from build123d import *

# Parameters (mm, degrees)
F0_W     = 70
F0_H     = 70
F0_R     = 1.1
F0_R_2   = 5.75
F1_DEPTH = 1.5
F3_DEPTH = 1.5


with BuildPart() as f1:
    # F0 (on Top) → F1 (new body)
    with BuildSketch(Plane.XY):
        Rectangle(F0_W, F0_H)
        with Locations((-20.071068, -5.384776)):
            Circle(F0_R, mode=Mode.SUBTRACT)
        with Locations((-31.384776, 5.928932)):
            Circle(F0_R, mode=Mode.SUBTRACT)
        with Locations((-4.868272, 21.131728)):
            Circle(F0_R_2, mode=Mode.SUBTRACT)
        with Locations((-5.928932, 31.384776)):
            Circle(F0_R, mode=Mode.SUBTRACT)
        with Locations((5.384776, 20.071068)):
            Circle(F0_R, mode=Mode.SUBTRACT)
    extrude(amount=F1_DEPTH)

    # F2 (on face) → F3 (cut, through all)
    with BuildSketch(Plane.XY.offset(1.5)):
        Polygon((-35, 35), (-35, 6.556349), (-6.556349, 35), align=None)
        Polygon((-20.857864, -8.84062), (-35, 5.301515), (-35, -35), (-15, -35), (-15, -8.84062), align=None)
    extrude(amount=-F3_DEPTH, mode=Mode.SUBTRACT)


solid = f1.part
For this review, take the finished solid that the model builds, in its own axes (mm). A direction names the side the tool comes from. Give positions to 0.01 mm unless a question says otherwise; leave off trailing zeros. Order: outer loops, then holes, each group sorted by start corner. A loop starts at its lowest first (then second) coordinate and runs counter-clockwise, first axis right, second up. Notation, with made-up numbers: (8.25, 88) -> (37.25, 88) arc R25 cw to (37.25, 107) -> close; hole circle Ø5 at (0.25, 19). An arc over 180 degrees is marked (long way). Write item = value, one per line.
1) We need section A-A, the plane y = 24. Give the boundary of the cut face in (x, z).
Findings:
outline = (-17.56, 0) -> (-9.85, 0) -> (-9.85, 1.5) -> (-17.56, 1.5) -> close; (0.12, 0) -> (35, 0) -> (35, 1.5) -> (0.12, 1.5) -> close
2) We need section C-C, the plane y = -17.5. Give the boundary of the cut face in (x, z).
Findings:
outline = (-15, 0) -> (35, 0) -> (35, 1.5) -> (-15, 1.5) -> close
3) To check wall thickness, follow L1, parallel to X at y = 6, z = 0.75; L2, parallel to X at y = -25.5, z = 0.7; L3, parallel to Y at x = -9, z = 0.8. State the ranges of each line that lie inside material, in increasing order. Write a range as from..to.
Findings:
L1 = -35..-32.48, -30.29..35
L2 = -15..35
L3 = -35..17.13, 25.13..32.56
4) Insertion check: pin 1 (2 mm diameter, centred on x = -31.38, y = 5.93, fed in from +Z) (1 decimal); pin 2 (0.8 mm diameter, centred on y = -26, z = 1, fed in from -X). Each pin has a flat end and moves straight along its axis. Give the tip position at first contact, or say it passes through.
Findings:
pin_1 = through
pin_2 = -15
5) We need section B-B, the plane z = 1.25. Give the boundary of the cut face in (x, y), and give its area (3 significant figures).
Findings:
outline = (-35, 5.3) -> (-20.86, -8.84) -> (-15, -8.84) -> (-15, -35) -> (35, -35) -> (35, 35) -> (-6.56, 35) -> (-35, 6.56) -> close; hole circle Ø2.2 at (-31.38, 5.93); hole circle Ø2.2 at (-20.07, -5.38); hole circle Ø11.5 at (-4.87, 21.13); hole circle Ø2.2 at (-5.93, 31.38); hole circle Ø2.2 at (5.38, 20.07)
area = 3,750 mm^2
6) We need section D-D, the plane x = -22. Give the boundary of the cut face in (y, z).
Findings:
outline = (-7.7, 0) -> (19.56, 0) -> (19.56, 1.5) -> (-7.7, 1.5) -> close
7) Draft analysis for pull direction Y (two halves, no side actions). For faces 1 (the face through (-6.17, 30.31, 0.74)), 2 (the face through (-27.8, -1.9, 0.8)), 3 (the face through (14, 35, 1)), state which applies: pulls with the +Y half, pulls with the -Y half, needs draft (parallel to the pull), parting line crosses it, or undercut.
Findings:
face_1 = undercut
face_2 = pulls with the -Y half
face_3 = pulls with the +Y half
8) For faces 4 (the face through (-15, -22, 1)), 5 (the face through (35, 0, 1)), list the 3-axis set-ups (+Z, -Z, +X, -X, +Y, -Y) from which the entire face can be reached by the end or side of a thin tool; tool diameter is ignored.
Findings:
face_4 = +Z, -Z, -X, -Y
face_5 = +Z, -Z, +X, +Y, -Y
